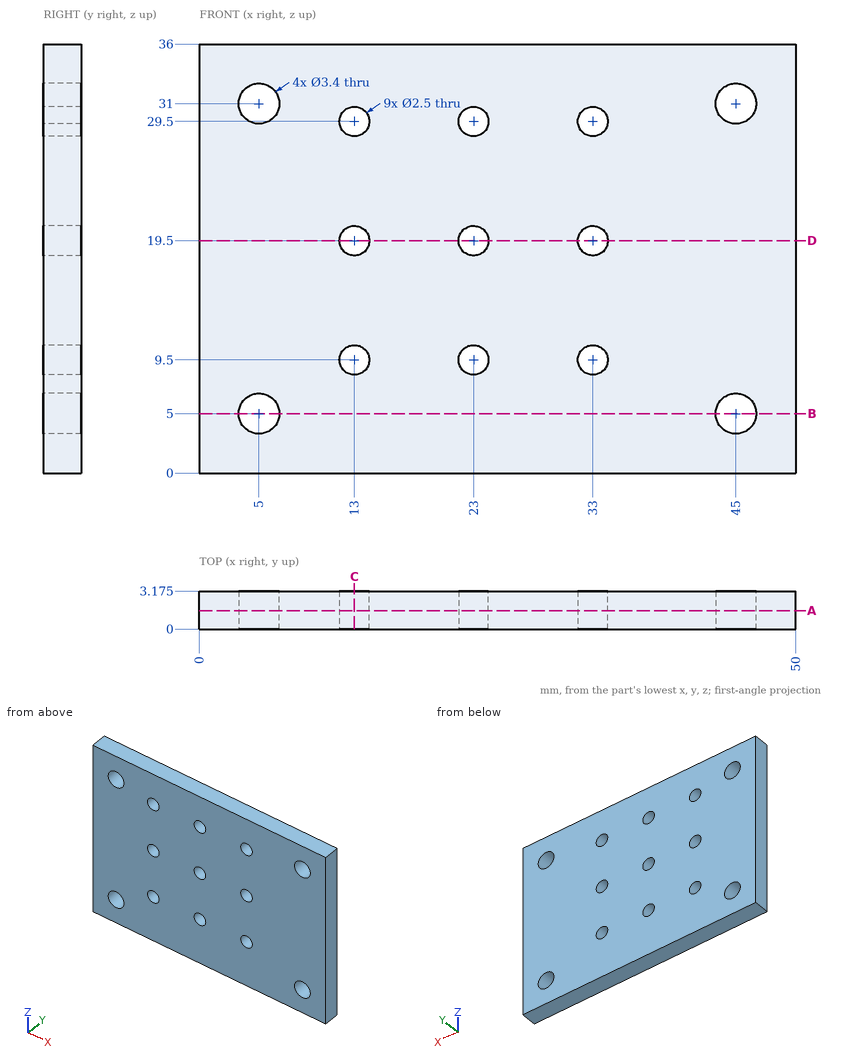
Study the drawing (mm; zero at the part's minimum x, y, z) and answer. Coordinates: 2 decimals unless noted, no trailing zeros. Write each loop counter-clockwise with the first axis right and the second up, starting at its lowest first coordinate (ties: lowest second). Pieces come first, ordered by that corner, then holes. Notation, with made-up numbers: (28, -5) - (83, -5) arc R19 ccw to (83, 27) - close; hole circle Ø5 at (34.5, 63). An arc over 180 degrees is marked (long way). One line per question, with ' | ' between items.
1) Find section C-C, the plane x = 13. Determine the outline of the cut face in (y, z) (3 decimals).
Checks:
outline: (0, 0) - (3.175, 0) - (3.175, 8.25) - (0, 8.25) - close; (0, 10.75) - (3.175, 10.75) - (3.175, 18.25) - (0, 18.25) - close; (0, 20.75) - (3.175, 20.75) - (3.175, 28.25) - (0, 28.25) - close; (0, 30.75) - (3.175, 30.75) - (3.175, 36) - (0, 36) - close
2) Consider probe 1 along Z at (x, y) = (5, 2.9); probe 2 along Z at (x, y) = (23, 2); probe 3 along X at (y, z) = (1.9, 9.5). Determine where each line is inside the solid, lowest interval first. Write a range as [from, to].
Checks:
probe 1: [0, 3.3], [6.7, 29.3], [32.7, 36] | probe 2: [0, 8.25], [10.75, 18.25], [20.75, 28.25], [30.75, 36] | probe 3: [0, 11.75], [14.25, 21.75], [24.25, 31.75], [34.25, 50]
3) A flat-ended cylindrical pin translates along its axis: P1, Ø2, axis at x = 13, z = 9.5, coming from the -Y side. Find the tip coordinate at first contact, or state that the pin passes through.
Checks:
P1: through
4) Find section D-D, the plane z = 19.5. Determine the outline of the cut face in (x, y) (3 decimals), and give its area (3 significant figures).
Checks:
outline: (0, 0) - (11.75, 0) - (11.75, 3.175) - (0, 3.175) - close; (14.25, 0) - (21.75, 0) - (21.75, 3.175) - (14.25, 3.175) - close; (24.25, 0) - (31.75, 0) - (31.75, 3.175) - (24.25, 3.175) - close; (34.25, 0) - (50, 0) - (50, 3.175) - (34.25, 3.175) - close | area: 135 mm2
5) Find section B-B, the plane z = 5. Determine the outline of the cut face in (x, y) (3 decimals).
Checks:
outline: (0, 0) - (3.3, 0) - (3.3, 3.175) - (0, 3.175) - close; (6.7, 0) - (43.3, 0) - (43.3, 3.175) - (6.7, 3.175) - close; (46.7, 0) - (50, 0) - (50, 3.175) - (46.7, 3.175) - close
6) Find section A-A, the plane y = 1.55. Give the number of separate pieces and of enclosed holes in the cut face, and give its area (3 significant figures).
Checks:
separate pieces: 1 | enclosed holes: 13 | area: 1,720 mm2
